The listing builds one solid part. Answer for the finished solid, in the listing's coordinates (mm). Face numbers are marked on the shaded views. A direction names the side the tool comes from. Coordinates: 2 decimals unless noted, no trailing zeros. Loops run counter-clockwise (first coordinate to the right, second up) from the corner with the lowest first, then second, coordinate; pieces in that order, holes last. Notation, with made-up numbers: (11.5, 9) - (55.5, 9) arc R13 ccw to (55.5, 19) - close; hole circle Ø10 at (23, 68.25). An arc over 180 degrees is marked (long way). Put each result on its own line as item: value.
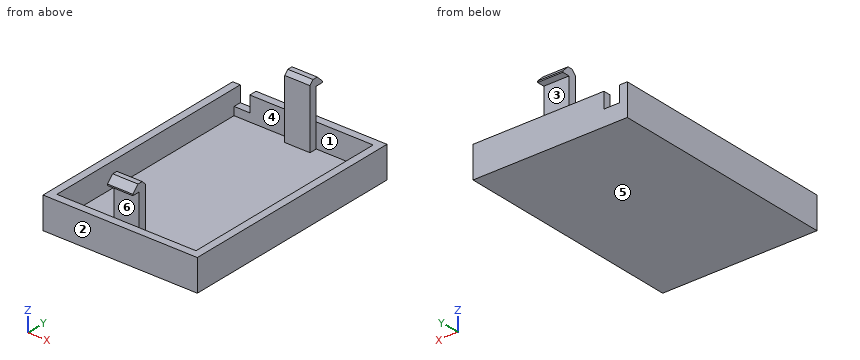
```python
from build123d import *

# Parameters (mm, degrees)
F0_W      = 22
F0_H      = 34
F1_DEPTH  = 1.2
F0_W_2    = 24.4
F0_H_2    = 36.4
F2_DEPTH  = 5
F3_W      = 4
F3_H      = 6.2
F3_H_2    = 3.8
F4_DEPTH  = 1.2
F5_SIZE   = 0.6
F6_W      = 4
F6_H      = 1.2
F7_DEPTH  = 1.2
F8_SIZE   = 1
F9_W      = 2.5
F9_H      = 2.5
F10_DEPTH = 25


# Not quite as in the source:
# - a pattern or mirror of a feature is missing from the dataset's text; its kind, count and spacing are read off the source's solid


with BuildPart() as f1:
    # F0 (on Top) → F1 (new body)
    with BuildSketch(Plane.XY):
        Rectangle(F0_W, F0_H)
    extrude(amount=F1_DEPTH)

    # F0 (on Top) → F2 (join)
    with BuildSketch(Plane.XY):
        Rectangle(F0_W_2, F0_H_2)
        Rectangle(F0_W, F0_H, mode=Mode.SUBTRACT)
    extrude(amount=F2_DEPTH)

    # F3 (on face) → F4 (join)
    with BuildSketch(Plane(origin=(0, -17, 0), x_dir=(-1, 0, 0), z_dir=(0, 1, 0))):
        with Locations((0, 8.1)):
            Rectangle(F3_W, F3_H)
        with Locations((0, 3.1)):
            Rectangle(F3_W, F3_H_2)
    f4 = extrude(amount=F4_DEPTH)

    # F4_copies: F4 across plane
    add(f4.mirror(Plane.ZX))

    # F5
    f5_edges = [f1.edges().sort_by_distance(p)[0] for p in [
        (0, -15.8, 11.2),
        (0, 15.8, 11.2),
    ]]
    chamfer(f5_edges, length=F5_SIZE)

    # F6 (on face) → F7 (join)
    with BuildSketch(Plane.XZ.offset(17)):
        with Locations((0, 10.6)):
            Rectangle(F6_W, F6_H)
    f7 = extrude(amount=F7_DEPTH)

    # F7_copies: F7 across plane
    add(f7.mirror(Plane.ZX))

    # F8
    f8_edges = [f1.edges().sort_by_distance(p)[0] for p in [
        (0, -18.2, 11.2),
        (0, 18.2, 11.2),
    ]]
    chamfer(f8_edges, length=F8_SIZE)

    # F9 (on face) → F10 (cut)
    with BuildSketch(Plane.XZ.offset(-17)):
        with Locations((-9.75, 3.75)):
            Rectangle(F9_W, F9_H)
    extrude(amount=-F10_DEPTH, mode=Mode.SUBTRACT)


solid = f1.part
```
1) The part is cut by section A-A (z = 8.5). Give the vertices of the cut face in (x, y).
Found:
outline: (-2, -17) - (2, -17) - (2, -15.8) - (-2, -15.8) - close; (-2, 15.8) - (2, 15.8) - (2, 17) - (-2, 17) - close
2) The part is cut by section C-C (z = 4). Give the vertices of the cut face in (x, y), and give its area (3 significant figures).
Found:
outline: (-12.2, -18.2) - (12.2, -18.2) - (12.2, 18.2) - (-8.5, 18.2) - (-8.5, 17) - (-2, 17) - (-2, 15.8) - (2, 15.8) - (2, 17) - (11, 17) - (11, -17) - (2, -17) - (2, -15.8) - (-2, -15.8) - (-2, -17) - (-11, -17) - (-11, 18.2) - (-12.2, 18.2) - close
area: 147 mm^2
3) Straight lines are drawn through the part: L1, parallel to X at y = -15, z = 3.25; L2, parallel to Y at x = 7.75, z = 1.5; L3, parallel to Y at x = 0.5, z = 8. For each, find the intervals that lie inside material, in ascending order. Write a range as [from, to].
Found:
L1: x = [-12.2, -11], [11, 12.2]
L2: y = [-18.2, -17], [17, 18.2]
L3: y = [-17, -15.8], [15.8, 17]
4) Each of these flat-tipped pins is pushed along its axis until it touches: pin 1 (2 mm diameter, centred on y = 14.5, z = 9.5, fed in from +X); pin 2 (1.2 mm diameter, centred on y = 16.5, z = 8, fed in from +X); pin 3 (1.2 mm diameter, centred on x = 1, z = 7.5, fed in from -Y); pin 4 (2 mm diameter, centred on x = 1, z = 7, fed in from +Y). Where does it stop, or does it pass through?
Found:
pin 1: passes through
pin 2: stops at x = 2
pin 3: stops at y = -17
pin 4: stops at y = 17
5) The part is cut by section D-D (y = 1). Give the vertices of the cut face in (x, z).
Found:
outline: (-12.2, 0) - (12.2, 0) - (12.2, 5) - (11, 5) - (11, 1.2) - (-11, 1.2) - (-11, 5) - (-12.2, 5) - close
6) For the marked faces 1, 2 and 3, determine the directions among +Z, -Z, +X, -X, +Y, -Y from which every point of the face is accessible in a straight line to the end or side of a thin tool.
Found:
face 1: +Z
face 2: +Z, -Z, +X, -X, -Y
face 3: +X, -X, +Y
7) For a pull along Z with two mould halves and no side action, classify the marked faces 4, 5 and 6 as pulls with the +Z half, pulls with the -Z half, needs draft (parallel to the pull), parting line crosses it, or undercut.
Found:
face 4: needs draft
face 5: pulls with the -Z half
face 6: undercut
8) The part is cut by section B-B (x = 7.5). Give the vertices of the cut face in (y, z).
Found:
outline: (-18.2, 0) - (18.2, 0) - (18.2, 5) - (17, 5) - (17, 1.2) - (-17, 1.2) - (-17, 5) - (-18.2, 5) - close
